```python
from build123d import *

# Parameters (mm, degrees)
SKETCH_R        = 15.159247
PAD_DEPTH       = 20
SKETCH001_R     = 8.82727
PAD001_DEPTH    = 13
SKETCH002_R     = 12.499133
POCKET_DEPTH    = 18
SKETCH003_R     = 6.812024
PAD002_DEPTH    = 60
POCKET001_DEPTH = 15


with BuildPart() as part:
    # Sketch → Pad (new body)
    with BuildSketch(Plane.XY):
        Circle(SKETCH_R)
    extrude(amount=PAD_DEPTH)

    # Sketch001 (on Face3 of Pad) → Pad001 (join)
    with BuildSketch(Plane.XY.offset(20)):
        Circle(SKETCH001_R)
    extrude(amount=PAD001_DEPTH)

    # Sketch002 (on Face2 of Pad001) → Pocket (cut)
    with BuildSketch(Plane(origin=(0, 0, 0), x_dir=(1, 0, 0), z_dir=(0, 0, -1))):
        Circle(SKETCH002_R)
    extrude(amount=-POCKET_DEPTH, mode=Mode.SUBTRACT)

    # Sketch003 (on Face6 of Pocket) → Pad002 (join)
    with BuildSketch(Plane(origin=(0, 0, 18), x_dir=(1, 0, 0), z_dir=(0, 0, -1))):
        Circle(SKETCH003_R)
    extrude(amount=PAD002_DEPTH)

    # Sketch004 (on Face9 of Pad002) → Pocket001 (cut)
    with BuildSketch(Plane(origin=(0, 0, -42), x_dir=(1, 0, 0), z_dir=(0, 0, -1))):
        with BuildLine():
            ThreePointArc((-3.949093, -1.795721), (0, -4.338197), (3.949093, -1.795721))
            Line((9.103818, -1.795721), (3.949093, -1.795721))
            Line((9.103818, 1.795721), (9.103818, -1.795721))
            Line((3.949093, 1.795721), (9.103818, 1.795721))
            ThreePointArc((3.949093, 1.795721), (0, 4.338197), (-3.949093, 1.795721))
            Line((-9.103818, 1.795721), (-3.949093, 1.795721))
            Line((-9.103818, -1.795721), (-9.103818, 1.795721))
            Line((-3.949093, -1.795721), (-9.103818, -1.795721))
        make_face()
    extrude(amount=-POCKET001_DEPTH, mode=Mode.SUBTRACT)


solid = part.part
```
CAD build for the part. Positions are in the model's coordinates, mm. A direction names the side the tool comes from. Round coordinates to 2 decimals unless told otherwise and drop trailing zeros. Write each loop counter-clockwise with the first axis right and the second up, starting at its lowest first coordinate (ties: lowest second). Pieces come first, ordered by that corner, then holes. Notation, with made-up numbers: (-32.5, 70) -> (-18.5, 70) arc R25 cw to (-18.5, 97) -> close; hole circle Ø8 at (86.5, -25.5). An arc over 180 degrees is marked (long way). Answer in a Markdown table with one row per item. Add a question column.
Item 1: Saw through at A-A, the plane z = -34. Write the cut outline in (x, y), then the cut area to 3 significant figures.
Item 2: Saw through at B-B, the plane y = 0. Write the cut outline in (x, z).
Item 3: Drop flat-ended pins along their axis: pin 1 Ø1.3 at (x, z) = (5.5, -32.5) entering from -Y; pin 2 Ø7 at (x, y) = (-0.5, 0) entering from -Z; pin 3 Ø10 at (y, z) = (10, -7.5) entering from -X. Give the stop position or say it passes through.
Item 4: Saw through at C-C, the plane z = 11. Write the cut outline in (x, y), then the cut area to 3 significant figures.
Item 5: Drill centre lines: line 1 (Y direction, x = 0, z = 13); line 2 (X direction, y = -6, z = 10.5); line 3 (X direction, y = -1, z = 7). Where is each one in solid material? Low to high. Write a range as from..to.
Item 6: Which spindle directions (+Z, -Z, +X, -X, +Y, -Y) get a long thin tool onto all of the face, cutting with end or side? Do faces 4 (the face through (-5, -1.796, -35)), 5 (the face through (0, 0, -27)), 6 (the face through (-12.03, -9.224, 9.86)), 7 (the face through (7, -7, 20)). Say none if no direction does.
Item 7: Saw through at D-D, the plane x = 0. Write the cut outline in (y, z), then the cut area to 3 significant figures.
Item 8: Mould opens along X. For faces 1 (the face through (5, 5, 18)), 2 (the face through (-1.91, -8.62, 26.41)), 3 (the face through (0, 5, -42)) say: pulls with the +X half, pulls with the -X half, needs draft (parallel to the pull), parting line crosses it, or undercut.
Findings below:
| question | item | result |
|---|---|---|
| 1 | outline | (-6.57, -1.8) arc R6.81 ccw to (6.57, -1.8) -> (3.95, -1.8) arc R4.34 cw to (-3.95, -1.8) -> close; (-6.57, 1.8) -> (-3.95, 1.8) arc R4.34 cw to (3.95, 1.8) -> (6.57, 1.8) arc R6.81 ccw to start |
| 1 | area | 68.5 mm^2 |
| 2 | outline | (-15.16, 0) -> (-12.5, 0) -> (-12.5, 18) -> (-6.81, 18) -> (-6.81, -27) -> (6.81, -27) -> (6.81, 18) -> (12.5, 18) -> (12.5, 0) -> (15.16, 0) -> (15.16, 20) -> (8.83, 20) -> (8.83, 33) -> (-8.83, 33) -> (-8.83, 20) -> (-15.16, 20) -> close |
| 3 | pin 1 | stops at y = -4.78 |
| 3 | pin 2 | stops at z = -27 |
| 3 | pin 3 | stops at x = -4.63 |
| 4 | outline | circle Ø30.32 at (0, 0); circle Ø13.62 at (0, 0); hole circle Ø25 at (0, 0) |
| 4 | area | 377 mm^2 |
| 5 | line 1 | y = -15.16..-12.5, -6.81..6.81, 12.5..15.16 |
| 5 | line 2 | x = -13.92..-10.96, -3.23..3.23, 10.96..13.92 |
| 5 | line 3 | x = -15.13..-12.46, -6.74..6.74, 12.46..15.13 |
| 6 | face 4 | -Z, +X, -X |
| 6 | face 5 | -Z |
| 6 | face 6 | +Z, -Z |
| 6 | face 7 | +Z |
| 7 | outline | (-15.16, 0) -> (-12.5, 0) -> (-12.5, 18) -> (-6.81, 18) -> (-6.81, -42) -> (-4.34, -42) -> (-4.34, -27) -> (4.34, -27) -> (4.34, -42) -> (6.81, -42) -> (6.81, 18) -> (12.5, 18) -> (12.5, 0) -> (15.16, 0) -> (15.16, 20) -> (8.83, 20) -> (8.83, 33) -> (-8.83, 33) -> (-8.83, 20) -> (-15.16, 20) -> close |
| 7 | area | 1,070 mm^2 |
| 8 | face 1 | undercut |
| 8 | face 2 | parting line crosses it |
| 8 | face 3 | needs draft |
